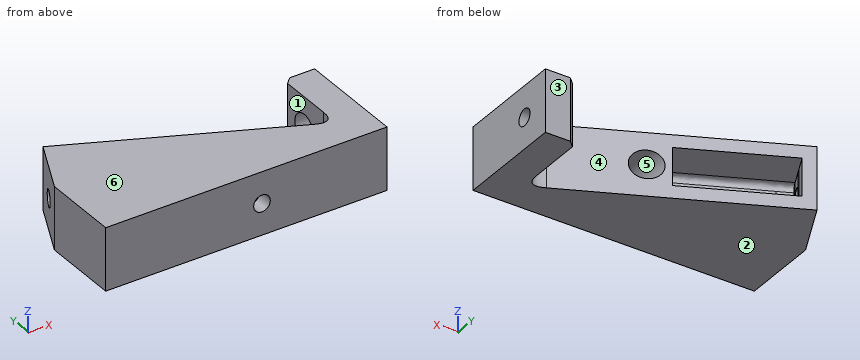
from build123d import *

# Parameters (mm, degrees)
BOSS_EXTRUDE2_DEPTH         = 12.7
CUT_EXTRUDE1_DEPTH          = 7.62
SKETCH3_R                   = 3.3
CUT_EXTRUDE3_DEPTH          = 5.08
FILLET1_START               = -124
FILLET1_DEPTH               = 45.095218809
FILLET1_START_2             = -7.62
FILLET1_2_DEPTH             = 16.62
FILLET1_3_DEPTH             = 46
F_1_4_CLEARANCE_HOLE1_D     = 6.7564
SKETCH8_R                   = 5.715
CUT_EXTRUDE4_DEPTH          = 137.313591586
CUT_EXTRUDE5_DEPTH          = 141.404698959
BOSS_EXTRUDE3_DEPTH         = 25.4
F_1_4_CLEARANCE_HOLE2_D     = 6.7564
F_1_4_CLEARANCE_HOLE2_DEPTH = 12.7
F_1_4_CLEARANCE_HOLE2_TIP   = 2.029827343
SKETCH14_R                  = 5.715
CUT_EXTRUDE6_DEPTH          = 6.604
CHAMFER1_SIZE               = 2.54


with BuildPart() as part:
    # Sketch1 → Boss-Extrude2 (new, symmetric)
    with BuildSketch(Plane.XY):
        Polygon((-127, 31.195273444), (-127, 0), (0, 0), (-116.265496152, 54.215491235), align=None)
    extrude(amount=BOSS_EXTRUDE2_DEPTH, both=True)

    # Sketch2 → Cut-Extrude1 (cut, symmetric)
    with BuildSketch(Plane.XY):
        Polygon((-115.634064254, 43.549297267), (-114.746565904, 45.45254362), (-109.127457625, 42.832310397), (-113.691734852, 33.044186297), (-119.310843131, 35.66441952), (-118.423344781, 37.567665873), align=None)
        Polygon((-71.512017628, 33.34660147), (-111.661452594, 52.068590465), (-114.746565904, 45.45254362), (-109.127457625, 42.832310397), (-113.691734852, 33.044186297), (-79.161408165, 16.942430525), align=None)
    extrude(amount=CUT_EXTRUDE1_DEPTH, both=True, mode=Mode.SUBTRACT)

    # Sketch3 → Cut-Extrude3 (cut)
    with BuildSketch(Plane(origin=(-116.265496152, 54.215491235, 0), x_dir=(0, 0, 1), z_dir=(-0.9063077870366528, 0.42261826174069317, 0))):
        with Locations(Location((0, -12.7, 0), (0, 0, 270))):
            Circle(SKETCH3_R)
    extrude(amount=-CUT_EXTRUDE3_DEPTH, mode=Mode.SUBTRACT)


with BuildPart() as fillet1_tool:
    # Fillet1: read off the stored shape, not the designer's step
    # Fillet1 outline → Fillet1 (new body)
    with BuildSketch(Plane(origin=(0, 0, 0), x_dir=(0.42261826174025074, 0.9063077870368592, -5.451523076012236e-13), z_dir=(0.9063077870368591, -0.42261826174025074, -1.1690828963840908e-12)).offset(FILLET1_START)):
        with BuildLine():
            Line((-18.1, 7.62), (-18.1, 5.08))
            add(Edge.make_bspline(
                [(-15.56, 7.62), (-15.987223051, 7.62), (-16.414446102, 7.62), (-17.356051224, 7.437902524), (-17.917902524, 6.876051224), (-18.1, 5.934446102), (-18.1, 5.507223051), (-18.1, 5.08)],
                knots=[0, 0, 0, 0, 0, 0, 0.5, 0.5, 1, 1, 1, 1, 1, 1], degree=5))
            Line((-15.56, 7.62), (-18.1, 7.62))
        make_face()
    extrude(amount=FILLET1_DEPTH)


with BuildPart() as part_1:
    add(part.part)


with BuildPart() as part_2:
    # Fillet1: joined with fillet1_tool
    add(part_1.part.fuse(fillet1_tool.part, tol=0.00001))


with BuildPart() as fillet1_2_tool:
    # Fillet1 2 outline → Fillet1 2 (new body)
    with BuildSketch(Plane.XY.offset(FILLET1_START_2)):
        with BuildLine():
            Line((-79.161408165, 16.942430525), (-78.087957781, 19.244452304))
            add(Edge.make_bspline(
                [(-78.087957781, 19.244452304), (-78.268510044, 18.857256726), (-78.449062307, 18.470061148), (-79.012038188, 17.693634812), (-79.758697015, 17.421873224), (-80.689038789, 17.654776383), (-81.076234367, 17.835328646), (-81.463429944, 18.015880909)],
                knots=[0, 0, 0, 0, 0, 0, 0.5, 0.5, 1, 1, 1, 1, 1, 1], degree=5))
            Line((-81.463429944, 18.015880909), (-79.161408165, 16.942430525))
        make_face()
    extrude(amount=FILLET1_2_DEPTH)


with BuildPart() as part_3:
    add(part_2.part)


with BuildPart() as part_4:
    # Fillet1 2: joined with fillet1_2_tool
    add(part_3.part.fuse(fillet1_2_tool.part, tol=0.00001))


with BuildPart() as fillet1_3_tool:
    # Fillet1 3 outline → Fillet1 3 (new body)
    with BuildSketch(Plane(origin=(0, 0, 0), x_dir=(0.42261826174025074, 0.9063077870368592, -5.451523076012236e-13), z_dir=(0.9063077870368591, -0.42261826174025074, -1.1690828963840908e-12)).offset(FILLET1_START)):
        with BuildLine():
            Line((-14, -7.62), (-15.56, -7.62))
            add(Edge.make_bspline(
                [(-15.56, -7.62), (-15.987223051, -7.62), (-16.414446102, -7.62), (-17.356051224, -7.437902524), (-17.917902524, -6.876051224), (-18.1, -5.934446102), (-18.1, -5.507223051), (-18.1, -5.08)],
                knots=[0, 0, 0, 0, 0, 0, 0.5, 0.5, 1, 1, 1, 1, 1, 1], degree=5))
            Line((-18.1, -5.08), (-18.1, -4))
            Line((-18.1, -4), (-20, -4))
            Line((-20, -4), (-20, -9))
            Line((-20, -9), (-14, -9))
            Line((-14, -9), (-14, -7.62))
        make_face()
    extrude(amount=FILLET1_3_DEPTH)


with BuildPart() as part_5:
    add(part_4.part)


with BuildPart() as part_6:
    # Fillet1 3: joined with fillet1_3_tool
    add(part_5.part.fuse(fillet1_3_tool.part, tol=0.00001))

    # 1/4 Clearance Hole1 (through all)
    with Locations(Plane(origin=(0, 0, 0), x_dir=(-1, 0, 0), z_dir=(0, -1, 0))):
        with Locations((63.5, 0)):
            Hole(F_1_4_CLEARANCE_HOLE1_D / 2)

    # Sketch8 → Cut-Extrude4 (cut, through all)
    with BuildSketch(Plane(origin=(0, 6.35, 0), x_dir=(-1, 0, 0), z_dir=(0, -1, 0))):
        with Locations(Location((63.5, 0, 0), (0, 0, 90))):
            Circle(SKETCH8_R)
    extrude(amount=-CUT_EXTRUDE4_DEPTH, mode=Mode.SUBTRACT)

    # Sketch9 → Cut-Extrude5 (cut, through all)
    with BuildSketch(Plane.XY.offset(12.7)):
        Polygon((-12.7, 5.922107259), (-12.7, 0), (0, 0), align=None)
    extrude(amount=-CUT_EXTRUDE5_DEPTH, mode=Mode.SUBTRACT)

    # Sketch10 → Boss-Extrude3 (add)
    with BuildSketch(Plane.XY.offset(12.7)):
        Polygon((-12.7, 5.922107259), (-12.7, 44.022107259), (-25.4, 44.022107259), (-25.4, 11.844214517), align=None)
    extrude(amount=-BOSS_EXTRUDE3_DEPTH)

    # 1/4 Clearance Hole2
    with Locations(Plane(origin=(-12.7, 0, 0), x_dir=(0, 0, -1), z_dir=(1, 0, 0))):
        with Locations((0, 31.322107259)):
            Hole(F_1_4_CLEARANCE_HOLE2_D / 2, depth=F_1_4_CLEARANCE_HOLE2_DEPTH)
            with Locations((0, 0, -(F_1_4_CLEARANCE_HOLE2_DEPTH + F_1_4_CLEARANCE_HOLE2_TIP / 2))):  # 118° drill point
                Cone(0, F_1_4_CLEARANCE_HOLE2_D / 2, F_1_4_CLEARANCE_HOLE2_TIP, mode=Mode.SUBTRACT)

    # Sketch14 → Cut-Extrude6 (cut)
    with BuildSketch(Plane.ZY.offset(25.4)):
        with Locations(Location((0, 31.322107259, 0), (0, 0, 270))):
            Circle(SKETCH14_R)
    extrude(amount=-CUT_EXTRUDE6_DEPTH, mode=Mode.SUBTRACT)

    # Chamfer1
    chamfer1_edges = [part_6.edges().sort_by_distance(p)[0] for p in [
        (-25.4, 44.022107259, 0),
    ]]
    chamfer(chamfer1_edges, length=CHAMFER1_SIZE)

    # Fillet2
    # a fillet whose section is not a circle: 5.08 mm, written as the material it adds along each edge (its section moved 0.00015 mm through the faces so that the kernel can cut it)
    with BuildSketch(Plane(origin=(-25.4, 11.844214517, 12.7), x_dir=(1.881112974510357e-05, 0.9999999998230706, 0), z_dir=(0, 0, -1))) as fillet2_piece_1:
        with BuildLine():
            add(Edge.make_bspline([(7.974002733, 0), (6.748845081, 2.3047e-05), (5.523687428, 4.6093e-05), (2.911264627, -0.681700719), (1.848095837, -2.35047216), (2.334181059, -5.00626823), (2.851934169, -6.11664789), (3.369687279, -7.227027551)], knots=[0, 0, 0, 0, 0, 0, 0.5, 0.5, 1, 1, 1, 1, 1, 1], degree=5))
            Line((3.369687279, -7.227027551), (3.277605601, -7.269963835))
            ThreePointArc((3.277605601, -7.269963835), (1.592829935, -3.656418364), (-0.092081679, -0.042936283))
            Line((-0.092081679, -0.042936283), (1.911e-06, 0.1016))
            ThreePointArc((1.911e-06, 0.1016), (3.987003276, 0.101525), (7.974004644, 0.1016))
            Line((7.974004644, 0.1016), (7.974002733, 0))
        make_face()
    extrude(amount=25.4)


solid = part_6.part
The model under review builds one solid part; all positions refer to its coordinate system, in mm. Face numbers are marked on the shaded views. A direction names the side the tool comes from. Round coordinates to 2 decimals unless told otherwise and drop trailing zeros. Write each loop counter-clockwise with the first axis right and the second up, starting at its lowest first coordinate (ties: lowest second). Pieces come first, ordered by that corner, then holes. Notation, with made-up numbers: M -9,74.5 L 3,74.5 A25 cw 3,94.5 Z; hole C -35,-7.75 d3. An arc over 180 degrees is marked long. Use a Markdown table: item, result. Add a question column.
Q1. We need section A-A, the plane x = -63.5. State the section outline as (y, z) points (3 decimals), plus the area to 3 significant figures.
Q2. The part is to be moulded in two halves that separate along Z. For the marked faces 4, 5 and 6, say which applies: pulls with the +Z half, pulls with the -Z half, needs draft (parallel to the pull), parting line crosses it, or undercut.
Q3. We need section B-B, the plane y = 22. Count the separate pieces of the cut face and the enclosed holes in it, plus the area to 3 significant figures.
Q4. Machinability: for the marked faces 1, 2 and 3, which of the approach directions +Z, -Z, +X, -X, +Y, -Y give a long, thin tool a straight path to every point of the face, cutting with its end or side? Answer none if there is none.
Q5. To check wall thickness, follow line 1 (Z direction, x = -83, y = 36.5); line 2 (X direction, y = 33, z = 6.75); line 3 (Y direction, x = -17.5, z = 0). State the ranges of each line that lie inside material, in increasing order.
Q6. Insertion check: pin 1 (2 mm diameter, centred on x = -84, z = 5.5, fed in from -Y); pin 2 (8 mm diameter, centred on y = 45, z = -7.5, fed in from -X); pin 3 (2 mm diameter, centred on x = -33, z = -7, fed in from +Y); pin 4 (8 mm diameter, centred on x = -51, z = -10, fed in from +Y). Each pin has a flat end and moves straight along its axis. Give the tip position at first contact, or say it passes through.
Findings below:
| question | item | result |
|---|---|---|
| 1 | outline | M 0,-12.7 L 29.611,-12.7 L 29.611,-5.715 L 6.35,-5.715 L 6.35,-3.378 L 0,-3.378 Z; M 0,3.378 L 6.35,3.378 L 6.35,5.715 L 29.611,5.715 L 29.611,12.7 L 0,12.7 Z |
| 1 | area | 443 mm² |
| 2 | face 4 | needs draft |
| 2 | face 5 | undercut |
| 2 | face 6 | pulls with the +Z half |
| 3 | separate pieces | 2 |
| 3 | enclosed holes | 2 |
| 3 | area | 2,050 mm² |
| 4 | face 1 | +Z, -Z, +Y |
| 4 | face 2 | -Z, +X, -X, +Y, -Y |
| 4 | face 3 | +Z, -Z, +X, +Y |
| 5 | line 1 | z = -12.7 to -7.62, 7.62 to 12.7 |
| 5 | line 2 | x = -126.16 to -112.84, -71.67 to -70.77, -25.4 to -12.7 |
| 5 | line 3 | y = 0 to 27.94, 34.7 to 44.02 |
| 6 | pin 1 | stops at y = 0 |
| 6 | pin 2 | stops at x = -122.43 |
| 6 | pin 3 | stops at y = 15.85 |
| 6 | pin 4 | stops at y = 25.65 |
